Can you work these out from the model? Positions are in its coordinate system, mm. A direction names the side the tool comes from. Give positions to 0.01 mm unless a question says otherwise; leave off trailing zeros. Order: outer loops, then holes, each group sorted by start corner. A loop starts at its lowest first (then second) coordinate and runs counter-clockwise, first axis right, second up. Notation, with made-up numbers: M 89.5,88 L 98.5,88 A35 cw 98.5,124 Z; hole C 77,66.25 d6. An arc over 180 degrees is marked long. Write each question's results on one line, items separated by ' | '.
from build123d import *

# Parameters (mm, degrees)
F0_W     = 410
F0_H     = 20
F0_W_2   = 20
F1_DEPTH = 498
F0_H_2   = 295
F2_DEPTH = 470
F3_DEPTH = 25


with BuildPart() as f1:
    # F0 (on Top) → F1 (new body)
    with BuildSketch(Plane.XY):
        with Locations((0, -157.5)):
            Rectangle(F0_W, F0_H)
        with Locations((-215, -157.5)):
            Rectangle(F0_W_2, F0_H)
        with Locations((215, -157.5)):
            Rectangle(F0_W_2, F0_H)
    extrude(amount=F1_DEPTH)

    # F0 (on Top) → F2 (join)
    with BuildSketch(Plane.XY):
        with Locations((-215, 0)):
            Rectangle(F0_W_2, F0_H_2)
        with Locations((-215, 157.5)):
            Rectangle(F0_W_2, F0_H)
        with Locations((0, 157.5)):
            Rectangle(F0_W, F0_H)
        with Locations((215, 157.5)):
            Rectangle(F0_W_2, F0_H)
        with Locations((215, 0)):
            Rectangle(F0_W_2, F0_H_2)
    extrude(amount=F2_DEPTH)

    # F0 (on Top) → F3 (join)
    with BuildSketch(Plane.XY):
        with Locations((215, -157.5)):
            Rectangle(F0_W_2, F0_H)
        with Locations((0, -157.5)):
            Rectangle(F0_W, F0_H)
        with Locations((215, 0)):
            Rectangle(F0_W_2, F0_H_2)
        with Locations((-215, -157.5)):
            Rectangle(F0_W_2, F0_H)
        with Locations((215, 157.5)):
            Rectangle(F0_W_2, F0_H)
        with Locations((-215, 0)):
            Rectangle(F0_W_2, F0_H_2)
        with Locations((0, 157.5)):
            Rectangle(F0_W, F0_H)
        with Locations((-215, 157.5)):
            Rectangle(F0_W_2, F0_H)
        Rectangle(F0_W, F0_H_2)
    extrude(amount=F3_DEPTH)


solid = f1.part
(1) Will these pins go through, and if not, where does the flat tip stop? P1, Ø6, axis at x = -30.5, y = 54.5, coming from the -Z side; P2, Ø1.5, axis at x = -23, y = 57.5, coming from the +Z side.
Data:
P1: stops at z = 0 | P2: stops at z = 25
(2) Imagine slicing it at C-C, the plane y = 42.5. Write out the boundary of the cut face in (x, z), plus the area to 4 significant figures.
Data:
outline: M -225,0 L 225,0 L 225,470 L 205,470 L 205,25 L -205,25 L -205,470 L -225,470 Z | area: 29,050 mm2
(3) Imagine slicing it at A-A, the plane x = -68. Write out the boundary of the cut face in (y, z), plus the area to 3 significant figures.
Data:
outline: M -167.5,0 L 167.5,0 L 167.5,470 L 147.5,470 L 147.5,25 L -147.5,25 L -147.5,498 L -167.5,498 Z | area: 26,700 mm2
(4) I need wall thicknesses on L1, parallel to Y at x = 204.5, z = 432.5; L2, parallel to X at y = 130, z = 331; L3, parallel to Z at x = 80, y = -77. Which ranges of each line are inside material? Lowest first, please. Write a range as from..to.
Data:
L1: y = -167.5..-147.5, 147.5..167.5 | L2: x = -225..-205, 205..225 | L3: z = 0..25
(5) We'd pull the mould along Y, two halves only. Please class faces 3 (the face through (205, -2, 244)), 4 (the face through (-3, 2, 25)), 5 (the face through (-18, 151, 470)), 6 (the face through (3, 167.5, 232)): +Y half, -Y half, draft (parallel to the pull), parting line (faces both ways), or undercut.
Data:
face 3: undercut | face 4: undercut | face 5: draft | face 6: +Y half
(6) For faces 1 (the face through (225, -2, 246)), 2 (the face through (-205, -2, 244)), which set-ups out of +Z, -Z, +X, -X, +Y, -Y let a thin tool reach every point of the face, with its end or its side?
Data:
face 1: +Z, -Z, +X, +Y, -Y | face 2: +Z
(7) Imagine slicing it at B-B, the plane z = 392. Write out the boundary of the cut face in (x, y), plus the area to 3 significant figures.
Data:
outline: M -225,-167.5 L 225,-167.5 L 225,167.5 L -225,167.5 Z; hole M -205,-147.5 L 205,-147.5 L 205,147.5 L -205,147.5 Z | area: 29,800 mm2
